The model under review builds one solid part; all positions refer to its coordinate system, in mm. A direction names the side the tool comes from. Coordinates: 2 decimals unless noted, no trailing zeros. Order: outer loops, then holes, each group sorted by start corner. A loop starts at its lowest first (then second) coordinate and runs counter-clockwise, first axis right, second up. Notation, with made-up numbers: (-36, 53) -> (-17, 53) arc R31 ccw to (-17, 84) -> close; hole circle Ø1 at (-28, -27.5). An arc over 180 degrees is marked (long way). Use one line per item in the form item = value.
from build123d import *

# Parameters (mm, degrees)
F1_DEPTH = 7
F2_DEPTH = 0.5
F3_SIZE  = 1.5


with BuildPart() as f1:
    # F0 (on Top) → F1 (new body)
    with BuildSketch(Plane.XY):
        with BuildLine():
            ThreePointArc((9.8694702636, -4.4606494482), (9.4166416974, -3.4255173739), (8.3699865077, -3))
            Line((8.3699865077, -3), (-8.0531213294, -3))
            ThreePointArc((-8.0531213294, -3), (-9.5065298079, -2.3739009406), (-10.0499606051, -0.8876037946))
            Line((-10.0499606051, -0.8876037946), (-9.9373864918, 1.1123962054))
            ThreePointArc((-9.9373864918, 1.1123962054), (-9.3144481567, 2.4534084785), (-7.9405472161, 3))
            Line((-7.9405472161, 3), (8.6688611699, 3))
            ThreePointArc((8.6688611699, 3), (9.7295213417, 3.4393398282), (10.1688611699, 4.5))
            ThreePointArc((10.1688611699, 4.5), (9.7295213417, 5.5606601718), (8.6688611699, 6))
            Line((8.6688611699, 6), (-10.8311388301, 6))
            ThreePointArc((-10.8311388301, 6), (-14.788404424, 2.0002282852), (-18.8302257154, 5.9145360656))
            ThreePointArc((-18.8302257154, 5.9145360656), (-19.5556040864, 5.3664207038), (-19.8311388301, 4.5))
            Line((-19.8311388301, 4.5), (-19.8311388301, -4.5))
            ThreePointArc((-19.8311388301, -4.5), (-19.6530330387, -5.2089398432), (-19.1610112284, -5.7495246306))
            ThreePointArc((-19.1610112284, -5.7495246306), (-15.0435619957, -2.001962967), (-11.1688611699, -6))
            Line((-11.1688611699, -6), (8.3699865077, -6))
            ThreePointArc((8.3699865077, -6), (9.4444691339, -5.5466551897), (9.8694702636, -4.4606494482))
        make_face()
        with BuildLine():
            ThreePointArc((-19.1610112284, -5.7495246306), (-15.2941603441, -9.998037033), (-11.1688611699, -6))
            Line((-11.1688611699, -6), (-13.1688611699, -6))
            ThreePointArc((-13.1688611699, -6), (-15.1688611699, -8), (-17.1688611699, -6))
            Line((-17.1688611699, -6), (-18.3311388301, -6))
            ThreePointArc((-18.3311388301, -6), (-18.7645630184, -5.9360165295), (-19.1610112284, -5.7495246306))
        make_face()
        with BuildLine():
            Line((-13.1688611699, -6), (-11.1688611699, -6))
            ThreePointArc((-11.1688611699, -6), (-15.0435619957, -2.001962967), (-19.1610112284, -5.7495246306))
            ThreePointArc((-19.1610112284, -5.7495246306), (-18.7645630184, -5.9360165295), (-18.3311388301, -6))
            Line((-18.3311388301, -6), (-17.1688611699, -6))
            ThreePointArc((-17.1688611699, -6), (-15.1688611699, -4), (-13.1688611699, -6))
        make_face()
        with BuildLine():
            ThreePointArc((-10.8311388301, 6), (-14.8738732362, 9.9997717148), (-18.8302257154, 5.9145360656))
            ThreePointArc((-18.8302257154, 5.9145360656), (-18.5843145611, 5.9784796411), (-18.3311388301, 6))
            Line((-18.3311388301, 6), (-16.8311388301, 6))
            ThreePointArc((-16.8311388301, 6), (-14.8311388301, 8), (-12.8311388301, 6))
            Line((-12.8311388301, 6), (-10.8311388301, 6))
        make_face()
        with BuildLine():
            ThreePointArc((-18.3311388301, 6), (-18.5843145611, 5.9784796411), (-18.8302257154, 5.9145360656))
            ThreePointArc((-18.8302257154, 5.9145360656), (-14.788404424, 2.0002282852), (-10.8311388301, 6))
            Line((-10.8311388301, 6), (-12.8311388301, 6))
            ThreePointArc((-12.8311388301, 6), (-14.8311388301, 4), (-16.8311388301, 6))
            Line((-16.8311388301, 6), (-18.3311388301, 6))
        make_face()
    extrude(amount=F1_DEPTH)

    # F0 (on Top) → F2 (join)
    with BuildSketch(Plane.XY):
        with BuildLine():
            ThreePointArc((9.8694702636, -4.4606494482), (9.4166416974, -3.4255173739), (8.3699865077, -3))
            Line((8.3699865077, -3), (-8.0531213294, -3))
            ThreePointArc((-8.0531213294, -3), (-9.5065298079, -2.3739009406), (-10.0499606051, -0.8876037946))
            Line((-10.0499606051, -0.8876037946), (-9.9373864918, 1.1123962054))
            ThreePointArc((-9.9373864918, 1.1123962054), (-9.3144481567, 2.4534084785), (-7.9405472161, 3))
            Line((-7.9405472161, 3), (8.6688611699, 3))
            ThreePointArc((8.6688611699, 3), (9.7295213417, 3.4393398282), (10.1688611699, 4.5))
            ThreePointArc((10.1688611699, 4.5), (9.7295213417, 5.5606601718), (8.6688611699, 6))
            Line((8.6688611699, 6), (-10.8311388301, 6))
            ThreePointArc((-10.8311388301, 6), (-14.788404424, 2.0002282852), (-18.8302257154, 5.9145360656))
            ThreePointArc((-18.8302257154, 5.9145360656), (-19.5556040864, 5.3664207038), (-19.8311388301, 4.5))
            Line((-19.8311388301, 4.5), (-19.8311388301, -4.5))
            ThreePointArc((-19.8311388301, -4.5), (-19.6530330387, -5.2089398432), (-19.1610112284, -5.7495246306))
            ThreePointArc((-19.1610112284, -5.7495246306), (-15.0435619957, -2.001962967), (-11.1688611699, -6))
            Line((-11.1688611699, -6), (8.3699865077, -6))
            ThreePointArc((8.3699865077, -6), (9.4444691339, -5.5466551897), (9.8694702636, -4.4606494482))
        make_face()
        with BuildLine():
            ThreePointArc((-19.1610112284, -5.7495246306), (-15.2941603441, -9.998037033), (-11.1688611699, -6))
            Line((-11.1688611699, -6), (-13.1688611699, -6))
            ThreePointArc((-13.1688611699, -6), (-15.1688611699, -8), (-17.1688611699, -6))
            Line((-17.1688611699, -6), (-18.3311388301, -6))
            ThreePointArc((-18.3311388301, -6), (-18.7645630184, -5.9360165295), (-19.1610112284, -5.7495246306))
        make_face()
        with BuildLine():
            Line((-13.1688611699, -6), (-11.1688611699, -6))
            ThreePointArc((-11.1688611699, -6), (-15.0435619957, -2.001962967), (-19.1610112284, -5.7495246306))
            ThreePointArc((-19.1610112284, -5.7495246306), (-18.7645630184, -5.9360165295), (-18.3311388301, -6))
            Line((-18.3311388301, -6), (-17.1688611699, -6))
            ThreePointArc((-17.1688611699, -6), (-15.1688611699, -4), (-13.1688611699, -6))
        make_face()
        with BuildLine():
            ThreePointArc((-10.8311388301, 6), (-14.8738732362, 9.9997717148), (-18.8302257154, 5.9145360656))
            ThreePointArc((-18.8302257154, 5.9145360656), (-18.5843145611, 5.9784796411), (-18.3311388301, 6))
            Line((-18.3311388301, 6), (-16.8311388301, 6))
            ThreePointArc((-16.8311388301, 6), (-14.8311388301, 8), (-12.8311388301, 6))
            Line((-12.8311388301, 6), (-10.8311388301, 6))
        make_face()
        with BuildLine():
            ThreePointArc((-18.3311388301, 6), (-18.5843145611, 5.9784796411), (-18.8302257154, 5.9145360656))
            ThreePointArc((-18.8302257154, 5.9145360656), (-14.788404424, 2.0002282852), (-10.8311388301, 6))
            Line((-10.8311388301, 6), (-12.8311388301, 6))
            ThreePointArc((-12.8311388301, 6), (-14.8311388301, 4), (-16.8311388301, 6))
            Line((-16.8311388301, 6), (-18.3311388301, 6))
        make_face()
        with BuildLine():
            Line((-16.8311388301, 6), (-12.8311388301, 6))
            ThreePointArc((-12.8311388301, 6), (-14.8311388301, 8), (-16.8311388301, 6))
        make_face()
        with BuildLine():
            ThreePointArc((-16.8311388301, 6), (-14.8311388301, 4), (-12.8311388301, 6))
            Line((-12.8311388301, 6), (-16.8311388301, 6))
        make_face()
        with BuildLine():
            Line((-17.1688611699, -6), (-13.1688611699, -6))
            ThreePointArc((-13.1688611699, -6), (-15.1688611699, -4), (-17.1688611699, -6))
        make_face()
        with BuildLine():
            ThreePointArc((-17.1688611699, -6), (-15.1688611699, -8), (-13.1688611699, -6))
            Line((-13.1688611699, -6), (-17.1688611699, -6))
        make_face()
    extrude(amount=-F2_DEPTH)

    # F3
    f3_edges = [f1.edges().sort_by_distance(p)[0] for p in [
        (-12.831139, 6, 7),
        (-17.168861, -6, 7),
    ]]
    chamfer(f3_edges, length=F3_SIZE)


solid = f1.part
Item 1: Clearance check with flat-ended pins moving along their axes: pin 1 (2.5 mm diameter, centred on x = -14.83, y = 6, fed in from +Z); pin 2 (1 mm diameter, centred on x = -3.5, z = 6, fed in from -Y); pin 3 (6 mm diameter, centred on x = -7.5, y = 8, fed in from +Z); pin 4 (1 mm diameter, centred on y = 0, z = 5, fed in from +X). State where each tip first meets the part, or that it passes through.
Results found:
pin_1 = 0
pin_2 = -6
pin_3 = 7
pin_4 = -9.97
Item 2: Tool access review of faces 1 (the face through (-6, 4, 7)), 2 (the face through (-15, -6, 0)): name each direction out of +Z, -Z, +X, -X, +Y, -Y from which nothing blocks a thin tool from reaching the whole face with its end or side.
Results found:
face_1 = +Z, +X, -X, +Y, -Y
face_2 = +Z
Item 3: We need section C-C (y = 0.5). Write out the cut boundary in (x, z), plus the area to 3 significant figures.
Results found:
outline = (-19.83, -0.5) -> (-9.97, -0.5) -> (-9.97, 7) -> (-19.83, 7) -> close
area = 73.9 mm²
Item 4: We need section A-A (x = -5.5). Write out the cut boundary in (y, z), plus the area to 3 significant figures.
Results found:
outline = (-6, -0.5) -> (-3, -0.5) -> (-3, 7) -> (-6, 7) -> close; (3, -0.5) -> (6, -0.5) -> (6, 7) -> (3, 7) -> close
area = 45.0 mm²
Item 5: Draft analysis for pull direction X (two halves, no side actions). For faces 3 (the face through (-17.167, -6.088, 2.712)), 4 (the face through (-12, 0, -0.5)), state which applies: released by +X, released by -X, zero draft, split by the parting line, or undercut.
Results found:
face_3 = undercut
face_4 = zero draft
Item 6: To check wall thickness, follow L1, parallel to Y at x = 5.5, z = 2.25; L2, parallel to X at y = -7.5, z = 2; L3, parallel to X at y = -5.5, z = 2.25. State the ranges of each line that lie inside material, in increasing order. Write a range as from..to.
Results found:
L1 = -6..-3, 3..6
L2 = -18.88..-16.49, -13.85..-11.46
L3 = -19.45..-17.11, -13.23..9.49
Item 7: We need section B-B (z = 0.75). Write out the cut boundary in (x, y).
Results found:
outline = (-19.83, -4.5) arc R1.5 ccw to (-19.16, -5.75) arc R4 ccw (long way) to (-11.17, -6) -> (8.37, -6) arc R1.5 ccw to (8.37, -3) -> (-8.05, -3) arc R2 cw to (-10.05, -0.89) -> (-9.94, 1.11) arc R2 cw to (-7.94, 3) -> (8.67, 3) arc R1.5 ccw to (8.67, 6) -> (-10.83, 6) arc R4 ccw (long way) to (-18.83, 5.91) arc R1.5 ccw to (-19.83, 4.5) -> close; hole circle Ø4 at (-15.17, -6); hole circle Ø4 at (-14.83, 6)
